from build123d import *

# Parameters (mm, degrees)
F1_DEPTH      = 12.7
F2_W          = 2.7
F2_H          = 12.7
F3_DEPTH      = 10
F4_R          = 3.5
F5_DEPTH      = 2.701
F5_DEPTH_BACK = 22.701
F6_T1_DEPTH   = 20.2
F7_W          = 8.7146805599
F7_H          = 16.2741800305
F8_DEPTH      = 5
F9_T1_DEPTH   = 16.8328947133
F9_T3_DEPTH   = 26.2954806011


# Not quite as in the source:
# - a fillet or chamfer that OpenCascade refuses, or shapes differently, is made with other operations: its cross-section is extruded or revolved along the edge and cut away or added


with BuildPart() as f1:
    # F0 (on Top) → F1 (new body)
    with BuildSketch(Plane.XY):
        with BuildLine():
            ThreePointArc((0, -12.7), (8.9802561211, -8.9802561211), (12.7, 0))
            ThreePointArc((12.7, 0), (0, 12.7), (-12.7, 0))
            Line((-12.7, 0), (-10, 0))
            ThreePointArc((-10, 0), (0, 10), (10, 0))
            ThreePointArc((10, 0), (7.0710678119, -7.0710678119), (0, -10))
            Line((0, -10), (0, -12.7))
        make_face()
    extrude(amount=F1_DEPTH)

    # F2 (on face) → F3 (join)
    with BuildSketch(Plane(origin=(0, 0, 0), x_dir=(0, -1, 0), z_dir=(-1, 0, 0))):
        with Locations((11.35, 6.35)):
            Rectangle(F2_W, F2_H)
    extrude(amount=F3_DEPTH)

    # F4 (on face) → F5 (cut, two sides)
    with BuildSketch(Plane(origin=(0, -10, 0), x_dir=(-1, 0, 0), z_dir=(0, 1, 0))) as f5_sk:
        with Locations((0, 6.35)):
            Circle(F4_R)
    extrude(amount=-F5_DEPTH, mode=Mode.SUBTRACT)
    extrude(f5_sk.sketch, amount=F5_DEPTH_BACK, mode=Mode.SUBTRACT)

    # F6: fillet of radius 1.5 on 2 edges, made by hand

    # F6_s2 → F6_t1 (cut)
    with BuildSketch(Plane.XY.offset(-3.75)):
        with BuildLine():
            ThreePointArc((-8.5, -10), (-9.5606601718, -10.4393398282), (-10, -11.5))
            Line((-10, -11.5), (-10, -10))
            Line((-10, -10), (-8.5, -10))
        make_face()
        with BuildLine():
            ThreePointArc((-8.5, -12.7), (-9.5606601718, -12.2606601718), (-10, -11.2))
            Line((-10, -11.2), (-10, -12.7))
            Line((-10, -12.7), (-8.5, -12.7))
        make_face()
    extrude(amount=F6_T1_DEPTH, mode=Mode.SUBTRACT)

    # F7 (on face) → F8 (cut)
    with BuildSketch(Plane.XZ):
        with Locations((-12.651483994, 6.0685008066)):
            Rectangle(F7_W, F7_H)
    extrude(amount=-F8_DEPTH, mode=Mode.SUBTRACT)

    # F9: fillet of radius 1.5 on 2 edges, made by hand

    # F9_s2 → F9_t1 (cut)
    with BuildSketch(Plane.XY.offset(-2.0664473567)):
        with BuildLine():
            ThreePointArc((-9.4868329805, 5), (-8.7874543743, 5.1730223946), (-8.249419983, 5.652173913))
            ThreePointArc((-8.249419983, 5.652173913), (-8.4611229501, 5.3300467562), (-8.6602540378, 5))
            Line((-8.6602540378, 5), (-9.4868329805, 5))
        make_face()
    extrude(amount=F9_T1_DEPTH, mode=Mode.SUBTRACT)

    # F9_s4 → F9_t3 (cut)
    with BuildSketch(Plane.XY.offset(-6.7977403006)):
        with BuildLine():
            ThreePointArc((-10.3423983333, 7.3705357143), (-10.4542350586, 5.812905964), (-9.1208552231, 5))
            Line((-9.1208552231, 5), (-11.6743308159, 5))
            ThreePointArc((-11.6743308159, 5), (-11.0719894554, 6.2210167577), (-10.3423983333, 7.3705357143))
        make_face()
    extrude(amount=F9_T3_DEPTH, mode=Mode.SUBTRACT)


solid = f1.part
Verification items for the finished model (mm, model axes). A direction names the side the tool comes from. Round coordinates to 2 decimals unless told otherwise and drop trailing zeros. Loops run counter-clockwise (first coordinate to the right, second up) from the corner with the lowest first, then second, coordinate; pieces in that order, holes last. Notation, with made-up numbers: (31.5, 25) - (38.5, 25) arc R14 ccw to (38.5, 34) - close; hole circle Ø7 at (-2.75, 88.25). An arc over 180 degrees is marked (long way). Use one line per item in the form item = value.
1. Section check A-A on z = 6.35. Record the cut outline in (x, y).
A:
outline = (-10.34, 7.37) arc R1.5 ccw to (-9.3, 5.01) arc R1.5 ccw to (-8.25, 5.65) arc R10 cw to (-3.5, 9.37) - (-3.5, 12.21) arc R12.7 ccw to start; (-9.99, -11.35) arc R1.5 ccw to (-8.5, -12.7) - (-3.5, -12.7) - (-3.5, -10) - (-8.5, -10) arc R1.5 ccw to start; (3.5, -12.21) arc R12.7 ccw to (3.5, 12.21) - (3.5, 9.37) arc R10 cw to (3.5, -9.37) - close
2. Access from +Z, -Z, +X, -X, +Y, -Y to the whole of each face (thin tool, end or side, straight path). Record for faces 1 (the cylindrical face through (-9.495, -10.377, 6.261)), 2 (the cylindrical face through (3.497, -11.381, 6.504)).
A:
face_1 = +Z, -Z, -X
face_2 = +Y, -Y
3. Draft check along X on faces 3 (the flat face through (11, 1, 12.7)), 4 (the cylindrical face through (-9.495, -12.323, 6.261)), 5 (the cylindrical face through (-8.72, 5.21, 6.26)), 6 (the cylindrical face through (-3.233, 11.014, 5.009)). Enter one of: pulls with the +X half, pulls with the -X half, needs draft (parallel to the pull), parting line crosses it, or undercut.
A:
face_3 = needs draft
face_4 = pulls with the -X half
face_5 = undercut
face_6 = undercut
4. Gauge pin test, flat ends, axial feed: pin 1 Ø7 at (x, z) = (-4, 6) entering from +Y; pin 2 Ø5 at (y, z) = (7.5, 3.5) entering from -X; pin 3 Ø1.5 at (x, z) = (9, 6.5) entering from +Y; pin 4 Ø1.5 at (y, z) = (2.5, 1.5) entering from -X. Record the tip position at first contact, or that the pin passes through.
A:
pin_1 = 12.58
pin_2 = -10.62
pin_3 = 9.66
pin_4 = 9.46
5. Section check D-D on z = 9.5. Record the cut outline in (x, y), and give its area (3 significant figures).
A:
outline = (-10.34, 7.37) arc R1.5 ccw to (-9.3, 5.01) arc R1.5 ccw to (-8.25, 5.65) arc R10 cw to (-1.53, 9.88) - (-1.53, 12.61) arc R12.7 ccw to start; (-9.99, -11.35) arc R1.5 ccw to (-8.5, -12.7) - (-1.53, -12.7) - (-1.53, -10) - (-8.5, -10) arc R1.5 ccw to start; (1.53, -12.61) arc R12.7 ccw to (1.53, 12.61) - (1.53, 9.88) arc R10 cw to (1.53, -9.88) - close
area = 138 mm²
6. Scan lines: probe 1 along Z at (x, y) = (0, 10.3); probe 2 along Z at (x, y) = (2.5, 10.25); probe 3 along X at (y, z) = (10.4, 6.35). Record each from-to range of solid material in increasing order.
A:
probe_1 = 0 to 2.85, 9.85 to 12.7
probe_2 = 0 to 3.9, 8.8 to 12.7
probe_3 = -7.29 to -3.5, 3.5 to 7.29
7. Section check C-C on x = -0.5. Record the cut outline in (y, z).
A:
outline = (-12.7, 0) - (-10, 0) - (-10, 2.89) - (-12.7, 2.89) - close; (-12.7, 9.81) - (-10, 9.81) - (-10, 12.7) - (-12.7, 12.7) - close; (9.99, 0) - (12.69, 0) - (12.69, 2.89) - (9.99, 2.89) - close; (9.99, 9.81) - (12.69, 9.81) - (12.69, 12.7) - (9.99, 12.7) - close
8. Section check B-B on x = -4.25. Record the cut outline in (y, z), and give its area (3 significant figures).
A:
outline = (-12.7, 0) - (-10, 0) - (-10, 12.7) - (-12.7, 12.7) - close; (9.05, 0) - (11.97, 0) - (11.97, 12.7) - (9.05, 12.7) - close
area = 71.3 mm²
